Here's how the part is built. I have some questions about the finished solid (model axes, mm). A direction names the side the tool comes from. Give positions to 0.01 mm unless a question says otherwise; leave off trailing zeros. Loops run counter-clockwise (first coordinate to the right, second up) from the corner with the lowest first, then second, coordinate; pieces in that order, holes last. Notation, with made-up numbers: (11, 37) - (44, 37) arc R16 cw to (44, 57) - close; hole circle Ø9 at (23, 34). An arc over 180 degrees is marked (long way). Return JSON: item names as keys, results as strings. Group by question number.
(1) I need wall thicknesses on probe 1 along Z at (x, y) = (1.25, 1); probe 2 along Y at (x, z) = (1.75, 19.05); probe 3 along Z at (x, y) = (3, 10). Which ranges of each line are inside material? Lowest first, please. Write a range as [from, to].
(2) On a 3-axis mill with a long thin cutter (end or side, diameter ignored), from which of +Z, -Z, +X, -X, +Y, -Y can I reach the whole of each face in a straight line? I mean faces 5 (the flat face through (7, 1, -21)), 6 (the flat face through (3, 12.75, 0)). Say none if no direction works.
(3) For P1, Ø2, axis at y = -6.72, z = -19.05, coming from the -X side; P2, Ø2, axis at x = 2.5, z = -64, coming from the -Y side; P3, Ø1.5, axis at x = 5, y = -78, coming from the -Z side; P4, Ø2, axis at x = 3, y = 4, coming from the -Z side, each with a flat end and sliding along its axis, tell me the tip position at first contact or that it passes through.
(4) If we section it at C-C (x = 3.5): State how many separate pieces and enclosed holes the cut face has, then the cut area to 3 significant figures.
(5) If we section it at D-D (y = -43): Please give me the cut outline in (x, z), then the cut area to 3 significant figures.
(6) If we section it at B-B (z = 0): Please give me the cut outline in (x, y), then the cut area to 3 significant figures.
(7) If we mould it in two halves opening along Z, with no side actions, what happens to faces 1 (the cylindrical face through (3.451, -99.184, 22.025)), 2 (the flat face through (3, -46.653, 0)), 3 (the flat face through (0, 1, -21)), 4 (the flat face through (3, -12.75, 0))? For each: released by +Z, released by -Z, zero draft, split by the parting line, or undercut.
(8) If we section it at A-A (y = 0): Please give me the cut outline in (x, z), then the cut area to 3 significant figures.
```python
from build123d import *

# Parameters (mm, degrees)
SKETCH1_R           = 101.6
SKETCH1_R_2         = 1.8
SKETCH1_W           = 25.5
SKETCH1_H           = 25.5
BOSS_EXTRUDE2_DEPTH = 7


with BuildPart() as part:
    # Sketch1 → Boss-Extrude2 (new body)
    with BuildSketch(Plane(origin=(0, 0, 0), x_dir=(0, 0, -1), z_dir=(1, 0, 0))):
        Circle(SKETCH1_R)
        with Locations((19.05, 6.718444761)):
            Circle(SKETCH1_R_2, mode=Mode.SUBTRACT)
        with Locations((19.05, -6.718444761)):
            Circle(SKETCH1_R_2, mode=Mode.SUBTRACT)
        with Locations((-6.718444761, -19.05)):
            Circle(SKETCH1_R_2, mode=Mode.SUBTRACT)
        with Locations((6.718444761, -19.05)):
            Circle(SKETCH1_R_2, mode=Mode.SUBTRACT)
        with Locations((-19.05, 6.718444761)):
            Circle(SKETCH1_R_2, mode=Mode.SUBTRACT)
        with Locations((-19.05, -6.718444761)):
            Circle(SKETCH1_R_2, mode=Mode.SUBTRACT)
        with Locations((6.718444761, 19.05)):
            Circle(SKETCH1_R_2, mode=Mode.SUBTRACT)
        with Locations((-6.718444761, 19.05)):
            Circle(SKETCH1_R_2, mode=Mode.SUBTRACT)
        Rectangle(SKETCH1_W, SKETCH1_H, mode=Mode.SUBTRACT)
        with BuildLine():
            Line((-19.05, -34.96193786), (19.05, -34.96193786))
            ThreePointArc((19.05, -34.96193786), (24.895725944, -40.807663805), (19.05, -46.653389749))
            Line((19.05, -46.653389749), (-19.05, -46.653389749))
            ThreePointArc((-19.05, -46.653389749), (-24.895725944, -40.807663805), (-19.05, -34.96193786))
        make_face(mode=Mode.SUBTRACT)
    extrude(amount=BOSS_EXTRUDE2_DEPTH)


solid = part.part
```
Values:
{
 "1": {"probe 1": "[-101.6, -12.75], [12.75, 101.6]", "probe 2": "[-99.8, -46.65], [-34.96, -8.52], [-4.92, 4.92], [8.52, 99.8]", "probe 3": "[-101.11, -12.75], [12.75, 101.11]"},
 "2": {"face 5": "+Z, -Z, +X, +Y, -Y", "face 6": "+X, -X"},
 "3": {"P1": "through", "P2": "y = -79.71", "P3": "z = -65.99", "P4": "z = -101.56"},
 "4": {"separate pieces": "1", "enclosed holes": "10", "area": "31,100 mm2"},
 "5": {"outline": "(0, -92.05) - (7, -92.05) - (7, -24.47) - (0, -24.47) - close; (0, 24.47) - (7, 24.47) - (7, 92.05) - (0, 92.05) - close", "area": "946 mm2"},
 "6": {"outline": "(0, -101.6) - (7, -101.6) - (7, -46.65) - (0, -46.65) - close; (0, -34.96) - (7, -34.96) - (7, -12.75) - (0, -12.75) - close; (0, 12.75) - (7, 12.75) - (7, 101.6) - (0, 101.6) - close", "area": "1,160 mm2"},
 "7": {"face 1": "split by the parting line", "face 2": "undercut", "face 3": "zero draft", "face 4": "undercut"},
 "8": {"outline": "(0, -101.6) - (7, -101.6) - (7, -12.75) - (0, -12.75) - close; (0, 12.75) - (7, 12.75) - (7, 101.6) - (0, 101.6) - close", "area": "1,240 mm2"}
}
